```python
from build123d import *

# Parameters (mm, degrees)
BOSS_EXTRUDE1_DEPTH = 10
SKETCH2_W           = 30
SKETCH2_H           = 20
CUT_EXTRUDE1_DEPTH  = 10
SKETCH3_R           = 10
BOSS_EXTRUDE2_DEPTH = 15


with BuildPart() as part:
    # Sketch1 → Boss-Extrude1 (new body)
    with BuildSketch(Plane(origin=(0, 0, 0), x_dir=(1, 0, 0), z_dir=(0, 1, 0))):
        with BuildLine():
            Line((30, -15), (-30, -15))
            ThreePointArc((-30, -15), (-45, 0), (-30, 15))
            Line((-30, 15), (30, 15))
            ThreePointArc((30, 15), (45, 0), (30, -15))
        make_face()
    extrude(amount=BOSS_EXTRUDE1_DEPTH)

    # Sketch2 → Cut-Extrude1 (cut)
    with BuildSketch(Plane(origin=(0, 10, 0), x_dir=(1, 0, 0), z_dir=(0, 1, 0))):
        Rectangle(SKETCH2_W, SKETCH2_H)
    extrude(amount=-CUT_EXTRUDE1_DEPTH, mode=Mode.SUBTRACT)

    # Sketch3 → Boss-Extrude2 (add)
    with BuildSketch(Plane(origin=(0, 10, 0), x_dir=(1, 0, 0), z_dir=(0, 1, 0))):
        with Locations(Location((-30, 0, 0), (0, 0, 270))):
            Circle(SKETCH3_R)
        with Locations(Location((30, 0, 0), (0, 0, 270))):
            Circle(SKETCH3_R)
    extrude(amount=BOSS_EXTRUDE2_DEPTH)


solid = part.part
```
Here's how the part is built. I have some questions about the finished solid (model axes, mm). A direction names the side the tool comes from. Round coordinates to 2 decimals unless told otherwise and drop trailing zeros. Order: outer loops, then holes, each group sorted by start corner. A loop starts at its lowest first (then second) coordinate and runs counter-clockwise, first axis right, second up. Notation, with made-up numbers: (14, -15) -> (31, -15) arc R14 cw to (31, 3) -> close; hole circle Ø2 at (65, -5). An arc over 180 degrees is marked (long way). Use a Markdown table: item, result. Add a question column.
(1) I need wall thicknesses on line 1 along Y through (x, z) = (31, -12.5); line 2 along Z through (x, y) = (-0.5, 8); line 3 along X through (y, z) = (13.5, 9). Which ranges of each line are inside material? Lowest first, please.
(2) Suppose I cut it at D-D, the plane y = 18.5. Please give me the cut outline in (x, z).
(3) If we mould it in two halves opening along X, with no side actions, what happens to faces 1 (the face through (-15, 5, 0)), 2 (the face through (20.24, 17.4, -2.17)), 3 (the face through (-30, 25, 0)), 4 (the face through (-45, 5, 0))? For each: released by +X, released by -X, zero draft, split by the parting line, or undercut.
(4) Suppose I cut it at A-A, the plane x = -9. Please give me the cut outline in (y, z), and give its area (3 significant figures).
(5) Suppose I cut it at C-C, the plane y = 4. Please give me the cut outline in (x, z).
(6) For faces 5 (the face through (0, 5, 10)), 6 (the face through (-39.76, 17.4, -2.17)), 7 (the face through (0.6, 0, -10.2)), which set-ups out of +Z, -Z, +X, -X, +Y, -Y let a thin tool reach every point of the face, with its end or its side?
(7) Suppose I cut it at B-B, the plane z = 0. Please give me the cut outline in (x, y).
(8) For pin 1 Ø1 at (y, z) = (18, 11.5) entering from -X; pin 2 Ø1 at (y, z) = (6.5, 1.5) entering from -X; pin 3 Ø8 at (x, z) = (10.5, -10.5) entering from +Y; pin 4 Ø6 at (y, z) = (4, 11) entering from -X, each with a flat end and sliding along its axis, tell me the tip position at first contact or that it passes through.
Verdict:
| question | item | result |
|---|---|---|
| 1 | line 1 | 0 to 10 |
| 1 | line 2 | -15 to -10, 10 to 15 |
| 1 | line 3 | -34.36 to -25.64, 25.64 to 34.36 |
| 2 | outline | circle Ø20 at (-30, 0); circle Ø20 at (30, 0) |
| 3 | face 1 | undercut |
| 3 | face 2 | undercut |
| 3 | face 3 | zero draft |
| 3 | face 4 | released by -X |
| 4 | outline | (0, -15) -> (10, -15) -> (10, -10) -> (0, -10) -> close; (0, 10) -> (10, 10) -> (10, 15) -> (0, 15) -> close |
| 4 | area | 100 mm2 |
| 5 | outline | (-30, -15) -> (30, -15) arc R15 ccw to (30, 15) -> (-30, 15) arc R15 ccw to start; hole (-15, -10) -> (15, -10) -> (15, 10) -> (-15, 10) -> close |
| 6 | face 5 | +Y, -Y |
| 6 | face 6 | +Y |
| 6 | face 7 | +Z, -Z, +X, -X, -Y |
| 7 | outline | (-45, 0) -> (-15, 0) -> (-15, 10) -> (-20, 10) -> (-20, 25) -> (-40, 25) -> (-40, 10) -> (-45, 10) -> close; (15, 0) -> (45, 0) -> (45, 10) -> (40, 10) -> (40, 25) -> (20, 25) -> (20, 10) -> (15, 10) -> close |
| 8 | pin 1 | through |
| 8 | pin 2 | x = -44.97 |
| 8 | pin 3 | y = 10 |
| 8 | pin 4 | x = -42.69 |
